Read the model definition and answer for the solid it produces. Units are mm, in the model's axes. A direction names the side the tool comes from. Coordinates: 2 decimals unless noted, no trailing zeros. Write each loop counter-clockwise with the first axis right and the second up, starting at its lowest first coordinate (ties: lowest second). Pieces come first, ordered by that corner, then holes. Notation, with made-up numbers: (-13, 58) - (13, 58) arc R25 cw to (13, 87) - close; hole circle Ø8 at (55.5, 89.25). An arc over 180 degrees is marked (long way). Return JSON: item names as keys, results as strings.
```python
from build123d import *

# Parameters (mm, degrees)
BOSS_EXTRUDE1_DEPTH = 6.35
CUT_EXTRUDE1_DEPTH  = 101.455184316


with BuildPart() as part:
    # Sketch1 → Boss-Extrude1 (new body)
    with BuildSketch(Plane.XY):
        Polygon((-30.233286112, -35.183650292), (-23.883286112, -35.183650292), (-23.883286112, -41.533650292), (40.404113888, -41.533650292), (40.404113888, -35.183650292), (46.754113888, -35.183650292), (46.754113888, -28.833650292), (53.104113888, -28.833650292), (53.104113888, 72.334549708), (46.754113888, 72.334549708), (46.754113888, 78.684549708), (40.404113888, 78.684549708), (40.404113888, 85.034549708), (-23.883286112, 85.034549708), (-23.883286112, 78.684549708), (-30.233286112, 78.684549708), (-30.233286112, 72.334549708), (-36.583286112, 72.334549708), (-36.583286112, -28.833650292), (-30.233286112, -28.833650292), align=None)
    extrude(amount=-BOSS_EXTRUDE1_DEPTH)

    # Sketch2 → Cut-Extrude1 (cut, through all)
    with BuildSketch(Plane(origin=(0, 0, -6.35), x_dir=(-1, 0, 0), z_dir=(0, 0, -1))):
        with BuildLine():
            Line((-20.668313863, 24.992906647), (-20.668313863, 18.507992769))
            ThreePointArc((-20.668313863, 18.507992769), (-35.451113888, 21.750449708), (-20.668313863, 24.992906647))
        make_face()
    extrude(amount=-CUT_EXTRUDE1_DEPTH, mode=Mode.SUBTRACT)


solid = part.part
```
(1) Straight lines are drawn through the part: line 1 (Y direction, x = -27, z = -3); line 2 (X direction, y = 22, z = -1.5); line 3 (Y direction, x = 48, z = -0.5). For each, find the intervals that lie inside material, in ascending order. Write a range as from..to.
Answer:
{"line 1": "-35.18..78.68", "line 2": "-36.58..20.67, 35.45..53.1", "line 3": "-28.83..72.33"}
(2) A cutting plane is placed at B-B (x = 22.5). Determine the outline of the cut face in (y, z), and give its area (3 significant figures).
Answer:
{"outline": "(-41.53, -6.35) - (16.01, -6.35) - (16.01, 0) - (-41.53, 0) - close; (27.49, -6.35) - (85.03, -6.35) - (85.03, 0) - (27.49, 0) - close", "area": "731 mm²"}
(3) A cutting plane is placed at C-C (y = 75). Determine the outline of the cut face in (x, z), and give its area (3 significant figures).
Answer:
{"outline": "(-30.23, -6.35) - (46.75, -6.35) - (46.75, 0) - (-30.23, 0) - close", "area": "489 mm²"}
(4) Which of the six approach directions +Z, -Z, +X, -X, +Y, -Y give full straight-line access (tool end or side, diameter ignored) to faces 1 (the face through (-30.233, -32, -3)), 2 (the face through (44, 78.685, -3)), 3 (the face through (-30.233, 76, -3))?
Answer:
{"face 1": "+Z, -Z, -X, -Y", "face 2": "+Z, -Z, +X, +Y", "face 3": "+Z, -Z, -X, +Y"}
(5) Flat-ended cylindrical pins translate along their axes: P1, Ø1.9, axis at y = -39, z = -3, coming from the -X side; P2, Ø3, axis at x = -26.5, z = -3.5, coming from the -Y side; P3, Ø1.9, axis at x = -27, z = -4.5, coming from the +Y side. Find the tip coordinate at first contact, or state that the pin passes through.
Answer:
{"P1": "x = -23.88", "P2": "y = -35.18", "P3": "y = 78.68"}
(6) Determine the mould class of faces 4 (the face through (8, 23, -6.35)), 5 (the face through (-27, -35.184, -3)), 6 (the face through (20.668, 22, -3)) for opening direction Y: +Y half, -Y half, draft (parallel to the pull), parting line (faces both ways), or undercut.
Answer:
{"face 4": "draft", "face 5": "-Y half", "face 6": "undercut"}
(7) A cutting plane is placed at A-A (z = -2.5). Determine the outline of the cut face in (x, y).
Answer:
{"outline": "(-36.58, -28.83) - (-30.23, -28.83) - (-30.23, -35.18) - (-23.88, -35.18) - (-23.88, -41.53) - (40.4, -41.53) - (40.4, -35.18) - (46.75, -35.18) - (46.75, -28.83) - (53.1, -28.83) - (53.1, 72.33) - (46.75, 72.33) - (46.75, 78.68) - (40.4, 78.68) - (40.4, 85.03) - (-23.88, 85.03) - (-23.88, 78.68) - (-30.23, 78.68) - (-30.23, 72.33) - (-36.58, 72.33) - close; hole (20.67, 18.51) arc R7.75 ccw (long way) to (20.67, 24.99) - close"}
(8) A cutting plane is placed at D-D (x = 33). Determine the outline of the cut face in (y, z).
Answer:
{"outline": "(-41.53, -6.35) - (16.1, -6.35) - (16.1, 0) - (-41.53, 0) - close; (27.4, -6.35) - (85.03, -6.35) - (85.03, 0) - (27.4, 0) - close"}
